Here's how the part is built. I have some questions about the finished solid (model axes, mm). Round coordinates to 2 decimals unless told otherwise and drop trailing zeros. Loops run counter-clockwise (first coordinate to the right, second up) from the corner with the lowest first, then second, coordinate; pieces in that order, holes last. Notation, with made-up numbers: M 39,59.5 L 50,59.5 A14 cw 50,86.5 Z; hole C 50.5,-18 d2. An arc over 180 degrees is marked long. Answer as a JSON object with one key per item and string values.
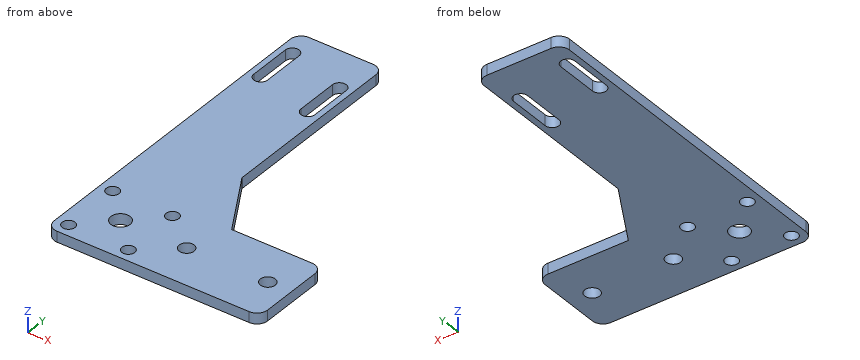
from build123d import *

# Parameters (mm, degrees)
ESQUISSE1_W                  = 40
ESQUISSE1_H                  = 160
BOSS_EXTRU_1_DEPTH           = 5
ENL_V_MAT_EXTRU_1_DEPTH      = 166
ENL_V_MAT_EXTRU_1_DEPTH_BACK = 166
ESQUISSE2_R                  = 4.5
ESQUISSE2_R_2                = 3
ESQUISSE3_W                  = 60
ESQUISSE3_H                  = 40
ESQUISSE3_R                  = 3.5
BOSS_EXTRU_2_DEPTH           = 5
CONG_1_R                     = 5
CHANFREIN1_SIZE              = 30
CHANFREIN1_SIZE2             = 17.320508076


with BuildPart() as part:
    # Esquisse1 → Boss.-Extru.1 (new body)
    with BuildSketch(Plane.XY):
        with Locations((20, 80)):
            Rectangle(ESQUISSE1_W, ESQUISSE1_H)
    extrude(amount=BOSS_EXTRU_1_DEPTH)

    # Esquisse2 → Enlèv. mat.-Extru.1 (cut, two sides: drawn at the far end of the back side and taken through both)
    with BuildSketch(Plane.XY.offset(5).offset(-ENL_V_MAT_EXTRU_1_DEPTH_BACK)):
        with Locations((20, 20)):
            Circle(ESQUISSE2_R)
        with Locations((6, 6)):
            Circle(ESQUISSE2_R_2)
        with Locations(Location((34, 6, 0), (0, 0, 180))):
            Circle(ESQUISSE2_R_2)
        with Locations((34, 34)):
            Circle(ESQUISSE2_R_2)
        with Locations(Location((6, 34, 0), (0, 0, 180))):
            Circle(ESQUISSE2_R_2)
        with BuildLine():
            Line((9.25, 148), (9.25, 128))
            ThreePointArc((9.25, 128), (6, 124.75), (2.75, 128))
            Line((2.75, 128), (2.75, 148))
            ThreePointArc((2.75, 148), (6, 151.25), (9.25, 148))
        make_face()
        with BuildLine():
            Line((30.75, 120), (30.75, 140))
            ThreePointArc((30.75, 140), (34, 143.25), (37.25, 140))
            Line((37.25, 140), (37.25, 120))
            ThreePointArc((37.25, 120), (34, 116.75), (30.75, 120))
        make_face()
    extrude(amount=ENL_V_MAT_EXTRU_1_DEPTH + ENL_V_MAT_EXTRU_1_DEPTH_BACK, mode=Mode.SUBTRACT)

    # Esquisse3 → Boss.-Extru.2 (add)
    with BuildSketch(Plane.XY.offset(5)):
        with Locations((70, 20)):
            Rectangle(ESQUISSE3_W, ESQUISSE3_H)
        with Locations((51, 20)):
            Circle(ESQUISSE3_R, mode=Mode.SUBTRACT)
        with Locations(Location((89, 20, 0), (0, 0, 180))):
            Circle(ESQUISSE3_R, mode=Mode.SUBTRACT)
    extrude(amount=-BOSS_EXTRU_2_DEPTH)

    # Congé1
    cong_1_edges = [part.edges().sort_by_distance(p)[0] for p in [
        (0, 160, 2.5),
        (40, 160, 2.5),
        (0, 0, 2.5),
        (100, 40, 2.5),
        (100, 0, 2.5),
    ]]
    fillet(cong_1_edges, radius=CONG_1_R)

    # Chanfrein1
    chanfrein1_edges = [part.edges().sort_by_distance(p)[0] for p in [
        (40, 40, 2.5),
    ]]
    chanfrein1_side = [part.faces().sort_by_distance(p)[0] for p in [
        (40, 97.5, 2.5),
    ]]
    chamfer(chanfrein1_edges, length=CHANFREIN1_SIZE, length2=CHANFREIN1_SIZE2, reference=chanfrein1_side[0])


solid = part.part
Item 1: I want a section at B-B, the plane z = 2.1. State how many separate pieces and enclosed holes the cut face has, then the cut area to 3 significant figures.
Resolved:
{"separate pieces": "1", "enclosed holes": "9", "area": "8,450 mm²"}
Item 2: I'm going to push flat-ended pins straight in: pin 1 Ø5.5 at (x, y) = (34, 6) entering from +Z; pin 2 Ø1.5 at (x, z) = (84.5, 1.5) entering from +Y; pin 3 Ø1.5 at (y, z) = (92.5, 3) entering from +X. Where does each tip first touch, or does it pass through?
Resolved:
{"pin 1": "through", "pin 2": "y = 40", "pin 3": "x = 40"}
Item 3: I want a section at D-D, the plane y = 85.5. Please give me the cut outline in (x, z), then the cut area to 3 significant figures.
Resolved:
{"outline": "M 0,0 L 40,0 L 40,5 L 0,5 Z", "area": "200 mm²"}
Item 4: Please list where these lines run through material, in increasing order: probe 1 along Y at (x, z) = (34, 2.8); probe 2 along X at (y, z) = (123, 4.3); probe 3 along Y at (x, z) = (20, 2.55). Write a range as from..to.
Resolved:
{"probe 1": "0..3, 9..31, 37..116.75, 143.25..160", "probe 2": "0..30.75, 37.25..40", "probe 3": "0..15.5, 24.5..160"}
Item 5: I want a section at C-C, the plane x = 20. Please give me the cut outline in (y, z), then the cut area to 3 significant figures.
Resolved:
{"outline": "M 0,0 L 15.5,0 L 15.5,5 L 0,5 Z; M 24.5,0 L 160,0 L 160,5 L 24.5,5 Z", "area": "755 mm²"}
Item 6: I want a section at A-A, the plane y = 20. Please give me the cut outline in (x, z), then the cut area to 3 significant figures.
Resolved:
{"outline": "M 0,0 L 15.5,0 L 15.5,5 L 0,5 Z; M 24.5,0 L 47.5,0 L 47.5,5 L 24.5,5 Z; M 54.5,0 L 85.5,0 L 85.5,5 L 54.5,5 Z; M 92.5,0 L 100,0 L 100,5 L 92.5,5 Z", "area": "385 mm²"}
